Input: dimensioned drawing with shaded views. Units: mm. Origin: part minimum x, y, z. A direction names the side the tool comes from. Round coordinates to 2 decimals unless told otherwise and drop trailing zeros. Write each loop counter-clockwise with the first axis right and the second up, starting at its lowest first coordinate (ties: lowest second). Pieces come first, ordered by that corner, then holes. Notation, with made-up numbers: M 67,-2 L 111,-2 A19 ccw 111,34 Z; hole C 18,38.5 d1. An arc over 180 degrees is marked long. Answer in a Markdown table with one row per item. Add a question column.
Item 1: Cut plane C-C on x = 102.5. Return loops of the section in (y, z).
Item 2: Material intervals for probe 1 along X at (y, z) = (3.3, 90); probe 2 along Z at (x, y) = (112.5, 3.5); probe 3 along Z at (x, y) = (37.5, 2), sorted ascending.
Item 3: Set-up query: the marked faces 4 and 5. Return all of +Z, -Z, +X, -X, +Y, -Y with unobstructed straight access to the full face (end or side cutting, diameter ignored); none if empty.
Item 4: Contact query for flat-ended pins moving along their axis: pin 1 (2 mm diameter, centred on x = 182.5, z = 90, fed in from -Y); pin 2 (1.5 mm diameter, centred on x = 122.5, z = 148, fed in from +Y). Output: stop coordinate, or through.
Item 5: Cut plane A-A on y = 20. Return loops of the section in (x, z), and give its area (4 significant figures).
Item 6: Mould query, pull axis X, two halves, no side actions, for the marked faces 1, 2 and 3. Classes: released by +X, released by -X, zero draft, split by the parting line, or undercut.
Item 7: Cut plane D-D on z = 223. Return loops of the section in (x, y).
Item 8: Cut plane B-B on z = 125. Return loops of the section in (x, y).
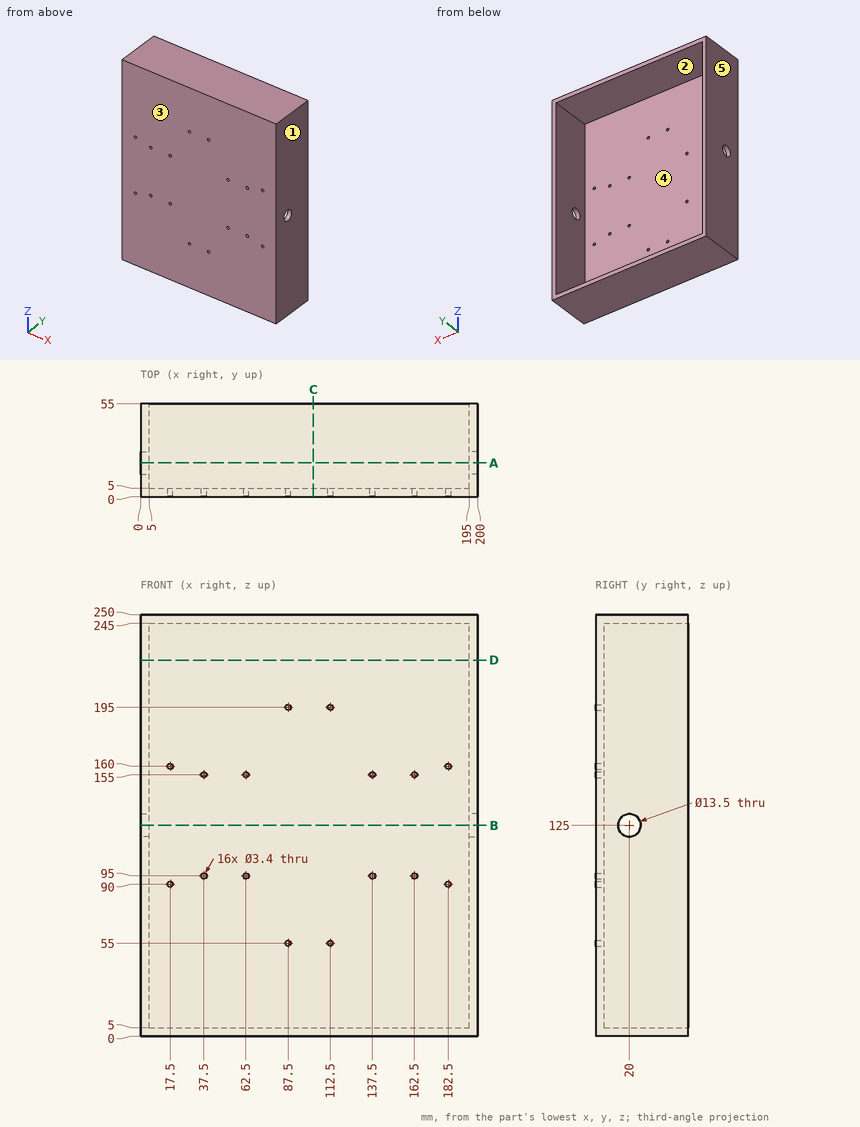
Results below:
| question | item | result |
|---|---|---|
| 1 | outline | M 0,0 L 55,0 L 55,5 L 5,5 L 5,245 L 55,245 L 55,250 L 0,250 Z |
| 2 | probe 1 | 0 to 15.8, 19.2 to 180.8, 184.2 to 200 |
| 2 | probe 2 | 0 to 53.3, 56.7 to 193.3, 196.7 to 250 |
| 2 | probe 3 | 0 to 93.3, 96.7 to 153.3, 156.7 to 250 |
| 3 | face 4 | +Y |
| 3 | face 5 | +Z, -Z, -X, +Y, -Y |
| 4 | pin 1 | through |
| 4 | pin 2 | y = 5 |
| 5 | outline | M 0,0 L 200,0 L 200,118.25 L 195,118.25 L 195,5 L 5,5 L 5,118.25 L 0,118.25 Z; M 0,131.75 L 5,131.75 L 5,245 L 195,245 L 195,131.75 L 200,131.75 L 200,250 L 0,250 Z |
| 5 | area | 4,265 mm2 |
| 6 | face 1 | released by +X |
| 6 | face 2 | undercut |
| 6 | face 3 | zero draft |
| 7 | outline | M 0,0 L 200,0 L 200,55 L 195,55 L 195,5 L 5,5 L 5,55 L 0,55 Z |
| 8 | outline | M 0,0 L 200,0 L 200,13.25 L 195,13.25 L 195,5 L 5,5 L 5,13.25 L 0,13.25 Z; M 0,26.75 L 5,26.75 L 5,55 L 0,55 Z; M 195,26.75 L 200,26.75 L 200,55 L 195,55 Z |
